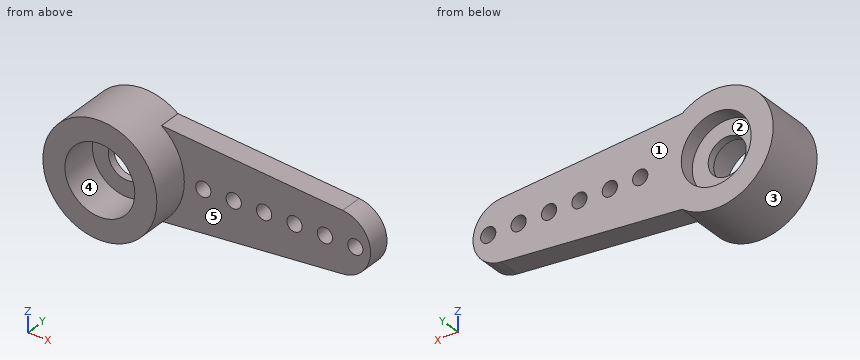
from build123d import *

# Parameters (mm, degrees)
SKETCH1_R           = 3.75
BOSS_EXTRUDE1_DEPTH = 4
SKETCH2_R           = 2.3
CUT_EXTRUDE1_DEPTH  = 1
SKETCH3_R           = 0.5
BOSS_EXTRUDE2_DEPTH = 1.5
SKETCH4_R           = 1.25
CUT_EXTRUDE2_DEPTH  = 4.5
SKETCH5_R           = 2.3
CUT_EXTRUDE3_DEPTH  = 2.5


with BuildPart() as part:
    # Sketch1 → Boss-Extrude1 (new body)
    with BuildSketch(Plane(origin=(0, 0, 0), x_dir=(1, 0, 0), z_dir=(0, 1, 0))):
        Circle(SKETCH1_R)
    extrude(amount=BOSS_EXTRUDE1_DEPTH)

    # Sketch2 → Cut-Extrude1 (cut)
    with BuildSketch(Plane(origin=(0, 4, 0), x_dir=(1, 0, 0), z_dir=(0, 1, 0))):
        Circle(SKETCH2_R)
    extrude(amount=-CUT_EXTRUDE1_DEPTH, mode=Mode.SUBTRACT)

    # Sketch3 → Boss-Extrude2 (add)
    with BuildSketch(Plane(origin=(0, 4, 0), x_dir=(1, 0, 0), z_dir=(0, 1, 0))):
        with BuildLine():
            Line((14.168399438, -1.992897797), (2.25, -3))
            ThreePointArc((2.25, -3), (3.75, 0), (2.25, 3))
            Line((2.25, 3), (14.168399438, 1.992897797))
            ThreePointArc((14.168399438, 1.992897797), (16, 0), (14.168399438, -1.992897797))
        make_face()
        with Locations((15, 0)):
            Circle(SKETCH3_R, mode=Mode.SUBTRACT)
        with Locations((5, 0)):
            Circle(SKETCH3_R, mode=Mode.SUBTRACT)
        with Locations((7, 0)):
            Circle(SKETCH3_R, mode=Mode.SUBTRACT)
        with Locations((9, 0)):
            Circle(SKETCH3_R, mode=Mode.SUBTRACT)
        with Locations((11, 0)):
            Circle(SKETCH3_R, mode=Mode.SUBTRACT)
        with Locations((13, 0)):
            Circle(SKETCH3_R, mode=Mode.SUBTRACT)
    extrude(amount=-BOSS_EXTRUDE2_DEPTH)

    # Sketch4 → Cut-Extrude2 (cut)
    with BuildSketch(Plane(origin=(0, 3, 0), x_dir=(1, 0, 0), z_dir=(0, 1, 0))):
        Circle(SKETCH4_R)
    extrude(amount=-CUT_EXTRUDE2_DEPTH, mode=Mode.SUBTRACT)

    # Sketch5 → Cut-Extrude3 (cut)
    with BuildSketch(Plane.XZ):
        Circle(SKETCH5_R)
    extrude(amount=-CUT_EXTRUDE3_DEPTH, mode=Mode.SUBTRACT)


solid = part.part
Here's how the part is built. I have some questions about the finished solid (model axes, mm). Face numbers are marked on the shaded views. A direction names the side the tool comes from. Give positions to 0.01 mm unless a question says otherwise; leave off trailing zeros. Loops run counter-clockwise (first coordinate to the right, second up) from the corner with the lowest first, then second, coordinate; pieces in that order, holes last. Notation, with made-up numbers: (58.25, -33.75) -> (113.25, -33.75) arc R20 cw to (113.25, 5.25) -> close; hole circle Ø9 at (37.5, -37.75). An arc over 180 degrees is marked (long way). One line per item, written item: value.
Q1. I'm going to push flat-ended pins straight in: pin 1 Ø2 at (x, z) = (10.5, -1) entering from -Y; pin 2 Ø2 at (x, z) = (0, 0) entering from +Y; pin 3 Ø1.5 at (y, z) = (1, 2.5) entering from -X; pin 4 Ø4 at (x, z) = (0, 0) entering from +Y. Where does each tip first touch, or does it pass through?
Answers follow:
pin 1: y = 2.5
pin 2: through
pin 3: x = -3.32
pin 4: y = 3
Q2. Suppose I cut it at A-A on y = 3.75. Please give me the cut outline in (x, z), then the cut area to 3 significant figures.
Answers follow:
outline: (2.25, -3) -> (14.17, -1.99) arc R2 ccw to (14.17, 1.99) -> (2.25, 3) arc R3.75 ccw (long way) to start; hole circle Ø4.6 at (0, 0); hole circle Ø1 at (5, 0); hole circle Ø1 at (7, 0); hole circle Ø1 at (9, 0); hole circle Ø1 at (11, 0); hole circle Ø1 at (13, 0); hole circle Ø1 at (15, 0)
area: 81.7 mm^2
Q3. On a 3-axis mill with a long thin cutter (end or side, diameter ignored), from which of +Z, -Z, +X, -X, +Y, -Y can I reach the whole of each face in a straight line? I mean the marked faces 1 and 2. Say none if no direction works.
Answers follow:
face 1: +Z, -Z, +X, -X, +Y
face 2: +Y
Q4. Suppose I cut it at B-B on x = 0. Please give me the cut outline in (y, z), then the cut area to 4 significant figures.
Answers follow:
outline: (0, -3.75) -> (4, -3.75) -> (4, -2.3) -> (3, -2.3) -> (3, -1.25) -> (2.5, -1.25) -> (2.5, -2.3) -> (0, -2.3) -> close; (0, 2.3) -> (2.5, 2.3) -> (2.5, 1.25) -> (3, 1.25) -> (3, 2.3) -> (4, 2.3) -> (4, 3.75) -> (0, 3.75) -> close
area: 12.65 mm^2
Q5. We'd pull the mould along X, two halves only. Please class the marked faces 3, 4 and 5: pulls with the +X half, pulls with the -X half, needs draft (parallel to the pull), parting line crosses it, or undercut.
Answers follow:
face 3: parting line crosses it
face 4: undercut
face 5: needs draft
Q6. Suppose I cut it at D-D on y = 1.55. Please give me the cut outline in (x, z).
Answers follow:
outline: circle Ø7.5 at (0, 0); hole circle Ø4.6 at (0, 0)
Q7. Suppose I cut it at C-C on z = 1. Please give me the cut outline in (x, y).
Answers follow:
outline: (-3.61, 0) -> (-2.07, 0) -> (-2.07, 2.5) -> (-0.75, 2.5) -> (-0.75, 3) -> (-2.07, 3) -> (-2.07, 4) -> (-3.61, 4) -> close; (0.75, 2.5) -> (2.07, 2.5) -> (2.07, 0) -> (3.61, 0) -> (3.61, 2.5) -> (15.73, 2.5) -> (15.73, 4) -> (2.07, 4) -> (2.07, 3) -> (0.75, 3) -> close
Q8. If I drill on line 1 along Z through (x, y) = (0, 3.2); line 2 along Z through (x, y) = (0, 2.85); line 3 along Y through (x, z) = (7.25, 2), over which ranges is the centre line in solid material (lowest first)?
Answers follow:
line 1: -3.75 to -2.3, 2.3 to 3.75
line 2: -3.75 to -1.25, 1.25 to 3.75
line 3: 2.5 to 4
